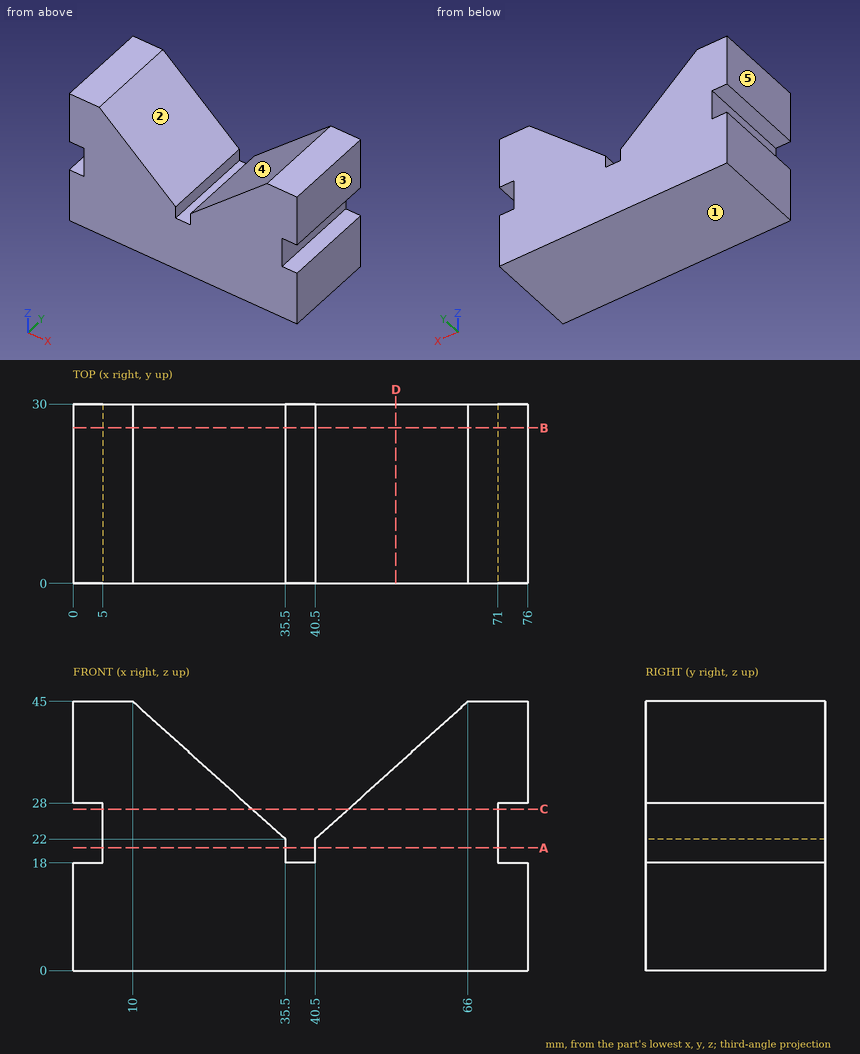
The figure shows three views and two pictorial views of one solid part (mm, origin at its lowest corner). Answer the questions. A direction names the side the tool comes from. Give positions to 0.01 mm unless a question says otherwise; leave off trailing zeros. Write each loop counter-clockwise with the first axis right and the second up, starting at its lowest first coordinate (ties: lowest second). Pieces come first, ordered by that corner, then holes. Notation, with made-up numbers: (69.25, 81) - (107.25, 81) arc R24 ccw to (107.25, 118) - close; hole circle Ø2 at (-21.5, 12). An arc over 180 degrees is marked (long way). Use one line per item in the form item = value.
1. A cutting plane is placed at B-B (y = 26). Write down the section's boundary in (x, z), and give its area (3 significant figures).
Filled in:
outline = (0, 0) - (76, 0) - (76, 18) - (71, 18) - (71, 28) - (76, 28) - (76, 45) - (66, 45) - (40.5, 22) - (40.5, 18) - (35.5, 18) - (35.5, 22) - (10, 45) - (0, 45) - (0, 28) - (5, 28) - (5, 18) - (0, 18) - close
area = 2,600 mm^2
2. Determine the mould class of the marked faces 3, 4 and 5 for opening direction X: released by +X, released by -X, zero draft, split by the parting line, or undercut.
Filled in:
face_3 = released by +X
face_4 = undercut
face_5 = released by -X
3. Each of these flat-tipped pins is pushed along its axis until it touches: pin 1 Ø1.5 at (y, z) = (23.5, 22.5) entering from -X; pin 2 Ø1.5 at (x, y) = (38, 12.5) entering from +Z; pin 3 Ø2 at (y, z) = (9.5, 19.5) entering from +X. Where does it stop, or does it pass through?
Filled in:
pin_1 = 5
pin_2 = 18
pin_3 = 71
4. A cutting plane is placed at D-D (x = 54). Write down the section's boundary in (y, z).
Filled in:
outline = (0, 0) - (30, 0) - (30, 34.18) - (0, 34.18) - close
5. A cutting plane is placed at A-A (z = 20.5). Write down the section's boundary in (x, y), and give its area (3 significant figures).
Filled in:
outline = (5, 0) - (35.5, 0) - (35.5, 30) - (5, 30) - close; (40.5, 0) - (71, 0) - (71, 30) - (40.5, 30) - close
area = 1,830 mm^2
6. A cutting plane is placed at C-C (z = 27). Write down the section's boundary in (x, y), and give its area (3 significant figures).
Filled in:
outline = (5, 0) - (29.96, 0) - (29.96, 30) - (5, 30) - close; (46.04, 0) - (71, 0) - (71, 30) - (46.04, 30) - close
area = 1,500 mm^2
7. Consider L1, parallel to X at y = 3.75, z = 21; L2, parallel to Z at x = 61, y = 10; L3, parallel to X at y = 26.5, z = 38.5. Determine where each line is inside the solid, lowest interval first.
Filled in:
L1 = 5 to 35.5, 40.5 to 71
L2 = 0 to 40.49
L3 = 0 to 17.21, 58.79 to 76
8. For the marked faces 1 and 2, determine the directions among +Z, -Z, +X, -X, +Y, -Y from which every point of the face is accessible in a straight line to the end or side of a thin tool.
Filled in:
face_1 = -Z, +X, -X, +Y, -Y
face_2 = +Z, +Y, -Y
